Geometry check sheet. Reference: the model listing, model coordinates, mm. A direction names the side the tool comes from. Round coordinates to 2 decimals unless told otherwise and drop trailing zeros. Order: outer loops, then holes, each group sorted by start corner. A loop starts at its lowest first (then second) coordinate and runs counter-clockwise, first axis right, second up.
```python
from build123d import *

# Parameters (mm, degrees)
SCHNITT_LINEAR_AUSTRAGEN1_DEPTH = 5.5


with BuildPart() as part:
    # Skizze1 → Rotation1 (revolve)
    with BuildSketch(Plane(origin=(0, 0, 0), x_dir=(0, 0, -1), z_dir=(1, 0, 0)), mode=Mode.PRIVATE) as rotation1_sk:
        Polygon((-6, 0), (-6, 5), (302.6, 5), (302.6, 12.5), (308.85, 12.5), (308.85, 0), align=None)
    revolve(rotation1_sk.sketch.rotate(Axis((0, 0, -308.85), (0, 0, 1)), 270), axis=Axis((0, 0, -308.85), (0, 0, 1)))

    # Skizze2 → Rotation2 (revolve)
    with BuildSketch(Plane(origin=(0, 0, 0), x_dir=(0, 0, -1), z_dir=(1, 0, 0)), mode=Mode.PRIVATE) as rotation2_sk:
        with BuildLine():
            Line((-28, 0), (-28, 4.233))
            Line((-28, 4.233), (-27.233, 5))
            Line((-27.233, 5), (-9.697981936, 5))
            Line((-9.697981936, 5), (-7.599415898, 4.236184428))
            ThreePointArc((-7.599415898, 4.236184428), (-7.498392718, 4.209115348), (-7.394203812, 4.2))
            Line((-7.394203812, 4.2), (-6.6, 4.2))
            ThreePointArc((-6.6, 4.2), (-6.175735931, 4.375735931), (-6, 4.8))
            Line((-6, 4.8), (-6, 5))
            Line((-6, 5), (-5, 5))
            Line((-5, 5), (-5, 0))
            Line((-5, 0), (-28, 0))
        make_face()
    revolve(rotation2_sk.sketch.rotate(Axis((0, 0, 5), (0, 0, 1)), 270), axis=Axis((0, 0, 5), (0, 0, 1)))

    # Skizze3 → Schnitt-Linear austragen1 (cut)
    with BuildSketch(Plane.XY.offset(1.5)):
        Polygon((-9, 18), (-9, -9), (-4.5, -9), (-4.5, 9), (4.5, 9), (4.5, -9), (9, -9), (9, 18), align=None)
    extrude(amount=SCHNITT_LINEAR_AUSTRAGEN1_DEPTH, mode=Mode.SUBTRACT)


solid = part.part
```
(1) Sectioned sample at C-C, the plane y = 9. Record the cut outline in (x, z).
Returned:
outline: (-8.67, -308.85) - (8.67, -308.85) - (8.67, -302.6) - (-8.67, -302.6) - close
(2) Set-up check for faces 1 (the flat face through (0.2, -5.4, -302.6)), 2 (the cylindrical face through (11.923, 3.755, -305.769)): record each of +Z, -Z, +X, -X, +Y, -Y from which the full face is reachable in a straight line by a thin tool's end or side.
Returned:
face 1: +Z
face 2: +Z, -Z
(3) Material ranges on line 1 (Z direction, x = 4, y = 10); line 2 (X direction, y = 0.75, z = -83.5); line 3 (Y direction, x = -0.5, z = -259), recorded low to high.
Returned:
line 1: z = -308.85 to -302.6
line 2: x = -4.94 to 4.94
line 3: y = -4.97 to 4.97
(4) Sectioned sample at B-B, the plane z = -261.5. Record the cut outline in (x, y).
Returned:
outline: circle Ø10 at (0, 0)
(5) Depth check by flat-ended pin: P1, Ø4, axis at x = 8.5, z = -14.5, coming from the -Y side; P2, Ø2, axis at y = 0, z = -48.5, coming from the -X side; P3, Ø1.5, axis at x = -5, y = 9, coming from the +Z side; P4, Ø3.5, axis at y = 0.5, z = 4.5, coming from the +X side. Enter the tip coordinate at first touch or a pass-through.
Returned:
P1: passes through
P2: stops at x = -5
P3: stops at z = -302.6
P4: stops at x = 4.5
(6) Sectioned sample at A-A, the plane x = 0. Record the cut outline in (y, z), and give its area (3 significant figures).
Returned:
outline: (-12.5, -308.85) - (12.5, -308.85) - (12.5, -302.6) - (5, -302.6) - (5, 6) - (4.8, 6) arc R0.6 cw to (4.2, 6.6) - (4.2, 7.39) arc R0.6 cw to (4.24, 7.6) - (5, 9.7) - (5, 27.23) - (4.23, 28) - (-4.23, 28) - (-5, 27.23) - (-5, 9.7) - (-4.24, 7.6) arc R0.6 cw to (-4.2, 7.39) - (-4.2, 6.6) arc R0.6 cw to (-4.8, 6) - (-5, 6) - (-5, -302.6) - (-12.5, -302.6) - close
area: 3,460 mm2
(7) Draft check along Z on faces 3 (the cylindrical face through (4.006, 1.262, 6.992)), 4 (the cylindrical face through (-1.08, -4.88, 18.34)), 5 (the flat face through (0, 0, 28)). Enter one of: released by +Z, released by -Z, zero draft, split by the parting line, or undercut.
Returned:
face 3: undercut
face 4: zero draft
face 5: released by +Z
